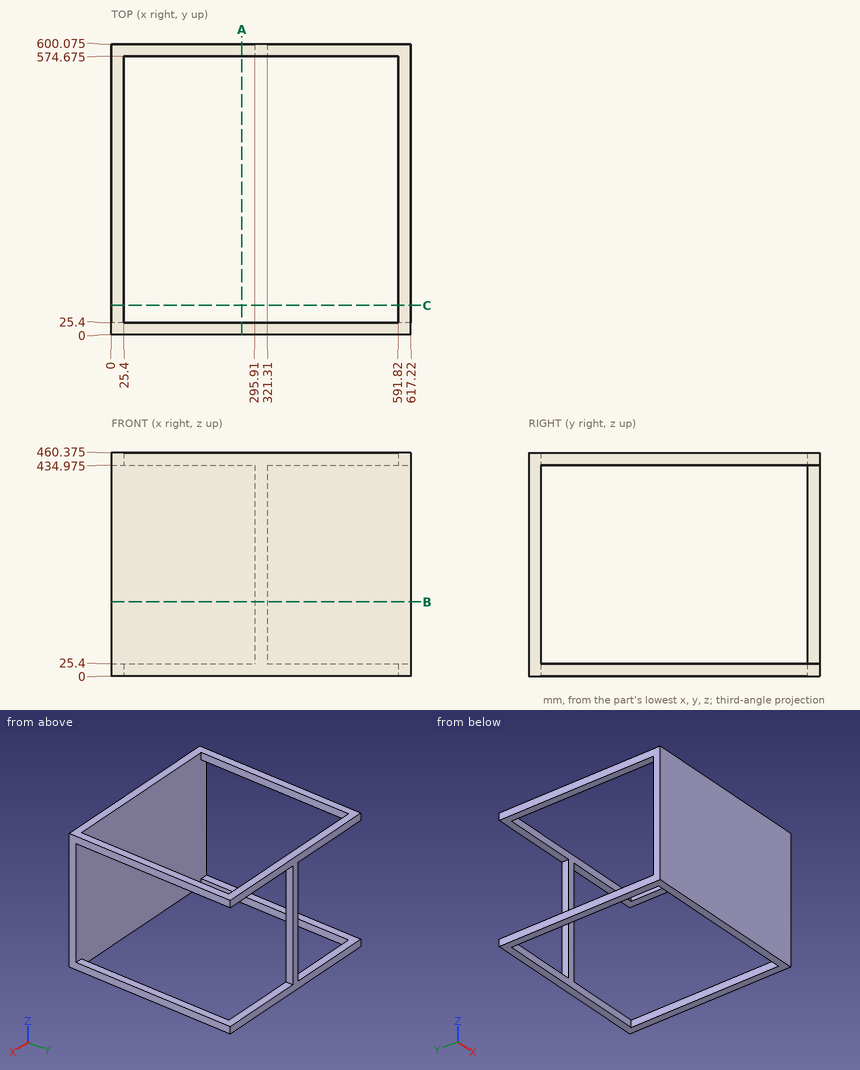
Geometry check sheet. Reference: drawing and pictorial views, mm from the part's lowest x, y, z. Round coordinates to 2 decimals unless told otherwise and drop trailing zeros. Loops run counter-clockwise (first coordinate to the right, second up) from the corner with the lowest first, then second, coordinate; pieces in that order, holes last. Notation, with made-up numbers: (45.25, 67) - (80.25, 67) arc R21 ccw to (80.25, 78) - close; hole circle Ø1 at (33.25, 21.25). An arc over 180 degrees is marked (long way). Write item = value, one per line. Start each with the question number.
Q1. Section check A-A (x = 269). Record the boundary of the cut face in (y, z) (3 decimals).
Q2. Thickness scan on L1, parallel to X at y = 269, z = 435.5; L2, parallel to Y at x = 310.5, z = 322 (3 decimals); L3, parallel to Y at x = 168, z = 100.5. Record the ranges inside material, lowest first.
Q3. Section check B-B (z = 153). Record the boundary of the cut face in (x, y) (3 decimals).
Q4. Depth check by flat-ended pin: P1, Ø12.5, axis at y = 288, z = 443, coming from the -X side; P2, Ø10, axis at x = 477, z = 215.5, coming from the +Y side; P3, Ø20.5, axis at y = 592, z = 257.5, coming from the +X side. Enter the tip coordinate at first touch or a pass-through.
Q5. Section check C-C (y = 61). Record the boundary of the cut face in (x, z) (3 decimals).
Derived:
q1.outline = (0, 0) - (25.4, 0) - (25.4, 460.375) - (0, 460.375) - close; (574.675, 0) - (600.075, 0) - (600.075, 25.4) - (574.675, 25.4) - close; (574.675, 434.975) - (600.075, 434.975) - (600.075, 460.375) - (574.675, 460.375) - close
q2.L1 = 0 to 25.4, 591.82 to 617.22
q2.L2 = 0 to 25.4, 574.675 to 600.075
q2.L3 = 0 to 25.4
q3.outline = (0, 0) - (617.22, 0) - (617.22, 25.4) - (0, 25.4) - close; (295.91, 574.675) - (321.31, 574.675) - (321.31, 600.075) - (295.91, 600.075) - close
q4.P1 = 0
q4.P2 = 25.4
q4.P3 = 321.31
q5.outline = (0, 0) - (25.4, 0) - (25.4, 25.4) - (0, 25.4) - close; (0, 434.975) - (25.4, 434.975) - (25.4, 460.375) - (0, 460.375) - close; (591.82, 0) - (617.22, 0) - (617.22, 25.4) - (591.82, 25.4) - close; (591.82, 434.975) - (617.22, 434.975) - (617.22, 460.375) - (591.82, 460.375) - close
